Verification items for the finished model (mm, model axes). Face numbers are marked on the shaded views. A direction names the side the tool comes from. Give positions to 0.01 mm unless a question says otherwise; leave off trailing zeros. Write each loop counter-clockwise with the first axis right and the second up, starting at its lowest first coordinate (ties: lowest second). Pieces come first, ordered by that corner, then holes. Notation, with made-up numbers: (86.25, 36) -> (95.25, 36) arc R17 ccw to (95.25, 51) -> close; hole circle Ø7 at (44.25, 88.25). An arc over 180 degrees is marked (long way). Answer as CSV lines item,"result".
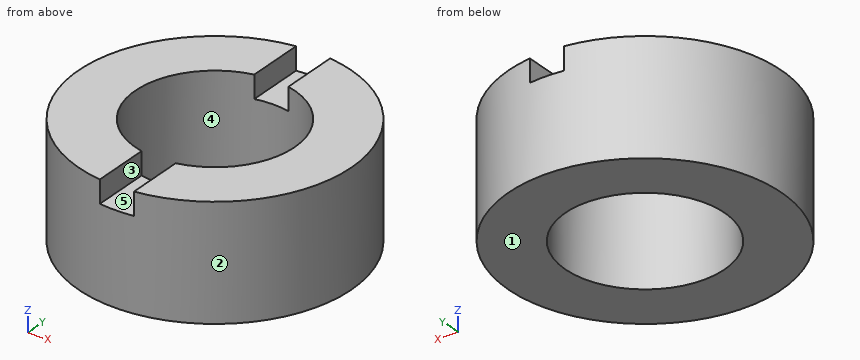
Autodesk Inventor part; units mm, degrees
ref_plane "YZ Plane" through (0, 0, 0) normal (1, 0, 0) x (0, 1, 0)
ref_plane "XZ Plane" through (0, 0, 0) normal (0, 1, 0) x (-1, 0, 0)
ref_plane "XY Plane" through (0, 0, 0) normal (0, 0, 1) x (1, 0, 0)
sketch "Sketch1" plane through (0, 0, 0) normal (0, 0, 1) x (1, 0, 0)
  circle A0 centre (0, 0) radius 6
  circle A1 centre (0, 0) radius 3.5
  dimension "d0" = 12
  dimension "d1" = 7
extrude "Extrusion1" add sketch "Sketch1" along normal blind 5
thread "Thread1"
sketch "Sketch2" plane through (0, 0, 5) normal (0, 0, 1) x (1, 0, 0)
  circle A0 centre (0, 0) radius 6
  line L0 (-0.75, 5.9529) -> (-0.75, -5.9529)
  line L1 (0.75, 5.9529) -> (0.75, -5.9529)
  line L2 (0, 0) -> (0, 6) construction
  dimension "d6" = 1.5
extrude "Extrusion2" cut sketch "Sketch2" against normal blind 1 contours L1 A0 L0
properties part number "37"
1) Depth check by flat-ended pin: pin 1 (1 mm diameter, centred on x = -1.5, z = 1, fed in from -Y); pin 2 (0.5 mm diameter, centred on x = 0, y = 4.5, fed in from +Z). Enter the tip coordinate at first touch or a pass-through.
Reported:
pin 1,"y = -5.92"
pin 2,"z = 4"
2) Tool access check on the marked faces 4 and 5. Record the directions out of +Z, -Z, +X, -X, +Y, -Y that give a thin tool (end or side, any length) a straight path to the whole face; none if there is none.
Reported:
face 4,"+Z, -Z"
face 5,"+Z, +Y, -Y"
3) Section check A-A (y = 0). Record the boundary of the cut face in (x, z).
Reported:
outline,"(-6, 0) -> (-3.5, 0) -> (-3.5, 5) -> (-6, 5) -> close; (3.5, 0) -> (6, 0) -> (6, 5) -> (3.5, 5) -> close"
4) Draft check along X on the marked faces 1, 2 and 3. Enter one of: +X half, -X half, draft (parallel to the pull), parting line (faces both ways), or undercut.
Reported:
face 1,"draft"
face 2,"parting line"
face 3,"undercut"
5) Scan lines: line 1 along X through (y, z) = (0.75, 4); line 2 along Y through (x, z) = (0, 3.2); line 3 along Y through (x, z) = (-1.25, 1.6). Record each from-to range of solid material in increasing order.
Reported:
line 1,"-5.95 to -3.42, 3.42 to 5.95"
line 2,"-6 to -3.5, 3.5 to 6"
line 3,"-5.87 to -3.27, 3.27 to 5.87"
6) Section check D-D (y = -3.75). Record the boundary of the cut face in (x, z), and give its area (3 significant figures).
Reported:
outline,"(-4.68, 0) -> (4.68, 0) -> (4.68, 5) -> (0.75, 5) -> (0.75, 4) -> (-0.75, 4) -> (-0.75, 5) -> (-4.68, 5) -> close"
area,"45.3 mm²"
7) Section check C-C (z = 3.35). Record the boundary of the cut face in (x, y).
Reported:
outline,"circle Ø12 at (0, 0); hole circle Ø7 at (0, 0)"
8) Section check B-B (x = 0). Record the boundary of the cut face in (y, z), and give its area (3 significant figures).
Reported:
outline,"(-6, 0) -> (-3.5, 0) -> (-3.5, 4) -> (-6, 4) -> close; (3.5, 0) -> (6, 0) -> (6, 4) -> (3.5, 4) -> close"
area,"20.0 mm²"
